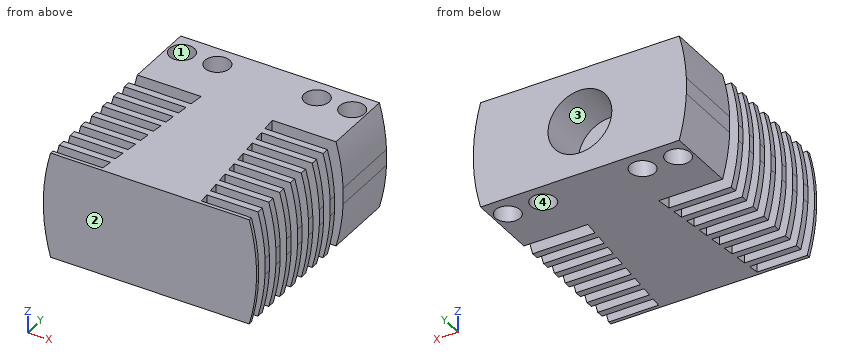
from build123d import *

# Parameters (mm, degrees)
SKETCH_1_W              = 30
SKETCH_1_H              = 30
EXTRUDE_1_DEPTH         = 15
HOLE_WIZARD_3_5_3_5_1_D = 3.5
CUT_EXTRUDE_1_DEPTH     = 46
CUT_EXTRUDE_2_REACH     = 47
SKETCH_6_R              = 4.5
CUT_EXTRUDE_3_DEPTH     = 7


with BuildPart() as part:
    # Эскиз1 → Бобышка-Вытянуть1 (new body)
    with BuildSketch(Plane.XY):
        with Locations((15, 15)):
            Rectangle(SKETCH_1_W, SKETCH_1_H)
    extrude(amount=EXTRUDE_1_DEPTH)

    # Диаметр отверстия Ø3.5 (3.5)1 (through all)
    with Locations(Plane.XY.offset(15)):
        with Locations((3, 27), (8, 27), (22, 27), (27, 27)):
            Hole(HOLE_WIZARD_3_5_3_5_1_D / 2)

    # Эскиз4 → Вырез-Вытянуть1 (cut, through all)
    with BuildSketch(Plane.XY.offset(15)):
        Polygon((0, 14.5), (9.45, 14.5), (9.3, 13), (0, 13), align=None)
        Polygon((0, 20), (10, 20), (9.8, 18), (0, 18), align=None)
        Polygon((0, 17), (9.7, 17), (9.55, 15.5), (0, 15.5), align=None)
        Polygon((0, 12), (9.2, 12), (9.05, 10.5), (0, 10.5), align=None)
        Polygon((0, 9.5), (8.95, 9.5), (8.8, 8), (0, 8), align=None)
        Polygon((0, 7), (8.7, 7), (8.55, 5.5), (0, 5.5), align=None)
        Polygon((0, 4.5), (8.45, 4.5), (8.3, 3), (0, 3), align=None)
        Polygon((0, 2), (8.2, 2), (8.05, 0.5), (0, 0.5), align=None)
        Polygon((21.8, 2), (21.95, 0.5), (30, 0.5), (30, 2), align=None)
        Polygon((21.55, 4.5), (21.7, 3), (30, 3), (30, 4.5), align=None)
        Polygon((21.3, 7), (21.45, 5.5), (30, 5.5), (30, 7), align=None)
        Polygon((21.05, 9.5), (21.2, 8), (30, 8), (30, 9.5), align=None)
        Polygon((20.8, 12), (20.95, 10.5), (30, 10.5), (30, 12), align=None)
        Polygon((20.55, 14.5), (20.7, 13), (30, 13), (30, 14.5), align=None)
        Polygon((20.3, 17), (20.45, 15.5), (30, 15.5), (30, 17), align=None)
        Polygon((30, 18), (20.2, 18), (20, 20), (30, 20), align=None)
    extrude(amount=-CUT_EXTRUDE_1_DEPTH, mode=Mode.SUBTRACT)

    # Вырез-Вытянуть2: up to this face of the body (flat: up to its plane)
    cut_extrude_2_end = Plane(part.part.faces().sort_by_distance((15, 0, 7.5))[0])
    # Эскиз5 → Вырез-Вытянуть2 (cut, up to the picked face)
    with BuildSketch(Plane(origin=(0, 30, 0), x_dir=(1, 0, 0), z_dir=(0, 1, 0)), mode=Mode.PRIVATE) as cut_extrude_2_sk1:
        with BuildLine():
            Line((30.335027773, 0), (30.335027773, -15))
            Line((30.335027773, -15), (29, -15))
            ThreePointArc((29, -15), (30.02315808, -7.5), (29, 0))
            Line((29, 0), (30.335027773, 0))
        make_face()
    cut_extrude_2_tool1 = split(extrude(cut_extrude_2_sk1.sketch, amount=-CUT_EXTRUDE_2_REACH, mode=Mode.PRIVATE), bisect_by=cut_extrude_2_end, keep=Keep.BOTH, mode=Mode.PRIVATE)
    # Эскиз5 → Вырез-Вытянуть2 (cut, up to the picked face)
    with BuildSketch(Plane(origin=(0, 30, 0), x_dir=(1, 0, 0), z_dir=(0, 1, 0)), mode=Mode.PRIVATE) as cut_extrude_2_sk2:
        with BuildLine():
            Line((-0.335027773, 0), (1, 0))
            ThreePointArc((1, 0), (-0.02315808, -7.5), (1, -15))
            Line((1, -15), (-0.335027773, -15))
            Line((-0.335027773, -15), (-0.335027773, 0))
        make_face()
    cut_extrude_2_tool2 = split(extrude(cut_extrude_2_sk2.sketch, amount=-CUT_EXTRUDE_2_REACH, mode=Mode.PRIVATE), bisect_by=cut_extrude_2_end, keep=Keep.BOTH, mode=Mode.PRIVATE)
    add(cut_extrude_2_tool1.solids().sort_by(Axis((29.667514, 30, 0.150593), (0, -1, 0)))[0], mode=Mode.SUBTRACT)
    add(cut_extrude_2_tool2.solids().sort_by(Axis((0.332486, 30, 14.849407), (0, -1, 0)))[0], mode=Mode.SUBTRACT)

    # Эскиз6 → Вырез-Вытянуть3 (cut)
    with BuildSketch(Plane(origin=(0, 30, 0), x_dir=(1, 0, 0), z_dir=(0, 1, 0))):
        with Locations(Location((15, -7.5, 0), (0, 0, 270))):
            Circle(SKETCH_6_R)
    extrude(amount=-CUT_EXTRUDE_3_DEPTH, mode=Mode.SUBTRACT)


solid = part.part
Work out the finished part from the listing and answer in its coordinate system (mm). Face numbers are marked on the shaded views. Coordinates: 2 decimals unless noted, no trailing zeros. Write each loop counter-clockwise with the first axis right and the second up, starting at its lowest first coordinate (ties: lowest second). Pieces come first, ordered by that corner, then holes. Notation, with made-up numbers: M 67,60.5 L 109,60.5 A20 ccw 109,66.5 Z; hole C 44,11.5 d5. An arc over 180 degrees is marked long. Use one line per item in the form item = value. Start each with the question number.
1. The part is cut by section B-B (x = 27). Give the number of separate pieces and of enclosed holes in the cut face, plus the area to 3 significant figures.
2. The part is cut by section A-A (y = 27). Give the vertices of the cut face in (x, z).
3. Straight lines are drawn through the part: probe 1 along X at (y, z) = (25.5, 12.5); probe 2 along Y at (x, z) = (21, 13.5); probe 3 along X at (y, z) = (23.5, 7). For each, find the intervals that lie inside material, in ascending order. Write a range as from..to.
4. The mould has two halves that part along Y. Classify the marked faces 1, 2, 3 and 4: released by +Y, released by -Y, zero draft, split by the parting line, or undercut.
Evaluation:
q1.separate_pieces = 10
q1.enclosed_holes = 0
q1.area = 210 mm^2
q2.outline = M 0,6.36 A28 ccw 1,0 L 1.25,0 L 1.25,15 L 1,15 A28 ccw 0,8.64 Z; M 4.75,0 L 6.25,0 L 6.25,15 L 4.75,15 Z; M 9.75,0 L 20.25,0 L 20.25,15 L 9.75,15 Z; M 23.75,0 L 25.25,0 L 25.25,15 L 23.75,15 Z; M 28.75,0 L 29,0 A28 ccw 30,6.36 L 30,8.64 A28 ccw 29,15 L 28.75,15 Z; hole C 15,7.5 d9
q3.probe_1 = 0.43..2.1, 3.9..7.1, 8.9..21.1, 22.9..26.1, 27.9..29.57
q3.probe_2 = 0..10.5, 12..13, 14.5..15.5, 17..18, 20..25.56, 28.44..30
q3.probe_3 = 0..10.53, 19.47..30
q4.face_1 = undercut
q4.face_2 = released by -Y
q4.face_3 = zero draft
q4.face_4 = undercut
